from build123d import *
from build123d.topology import SkipClean

# Parameters (mm, degrees)
SKETCH1_W           = 50
SKETCH1_H           = 60
BOSS_EXTRUDE1_DEPTH = 12
SKETCH2_W           = 41
SKETCH2_H           = 4.2
CUT_EXTRUDE1_DEPTH  = 67.098411479
SKETCH3_W           = 12
SKETCH3_H           = 30
BOSS_EXTRUDE2_DEPTH = 42
SKETCH4_W           = 7.2
SKETCH4_H           = 20
CUT_EXTRUDE2_DEPTH  = 42.5
SKETCH5_R           = 2.55
CUT_EXTRUDE3_DEPTH  = 35
FILLET1_R           = 5
SKETCH6_R           = 2.55
CUT_EXTRUDE4_DEPTH  = 35
SKETCH7_R           = 2.9
BOSS_EXTRUDE3_DEPTH = 5


with BuildPart() as part:
    # Sketch1 → Boss-Extrude1 (new body)
    with BuildSketch(Plane.XY):
        Rectangle(SKETCH1_W, SKETCH1_H)
    extrude(amount=BOSS_EXTRUDE1_DEPTH)

    # Sketch2 → Cut-Extrude1 (cut, through all)
    with BuildSketch(Plane(origin=(0, 30, 0), x_dir=(1, 0, 0), z_dir=(0, 1, 0))):
        with Locations((0, -8.9)):
            Rectangle(SKETCH2_W, SKETCH2_H)
    extrude(amount=-CUT_EXTRUDE1_DEPTH, mode=Mode.SUBTRACT)

    # Sketch3 → Boss-Extrude2 (add)
    with BuildSketch(Plane.ZY.offset(25)):
        with Locations((6, -15)):
            Rectangle(SKETCH3_W, SKETCH3_H)
    boss_extrude2 = extrude(amount=BOSS_EXTRUDE2_DEPTH)

    # Sketch4 → Cut-Extrude2 (cut)
    with BuildSketch(Plane.ZY.offset(67)):
        with Locations((7.4, -15)):
            Rectangle(SKETCH4_W, SKETCH4_H)
    cut_extrude2 = extrude(amount=-CUT_EXTRUDE2_DEPTH, mode=Mode.SUBTRACT)

    # Sketch5 → Cut-Extrude3 (cut)
    with BuildSketch(Plane.XY.offset(12)):
        with Locations((-59.5, -14.995756269)):
            Circle(SKETCH5_R)
        with Locations((-51.2, -14.995756269)):
            Circle(SKETCH5_R)
        with Locations((-42.9, -14.995756269)):
            Circle(SKETCH5_R)
        with Locations((-34.6, -14.995756269)):
            Circle(SKETCH5_R)
    cut_extrude3 = extrude(amount=-CUT_EXTRUDE3_DEPTH, mode=Mode.SUBTRACT)

    # Mirror1: Boss-Extrude2, Cut-Extrude2, Cut-Extrude3 across plane
    add(boss_extrude2.mirror(Plane(origin=(0, 0, 0), x_dir=(0, 0, 1), z_dir=(1, 0, 0))))
    add(cut_extrude2.mirror(Plane(origin=(0, 0, 0), x_dir=(0, 0, 1), z_dir=(1, 0, 0))), mode=Mode.SUBTRACT)
    add(cut_extrude3.mirror(Plane(origin=(0, 0, 0), x_dir=(0, 0, 1), z_dir=(1, 0, 0))), mode=Mode.SUBTRACT)

    # Fillet1
    # the kernel refuses this fillet: 5 mm, written as the material it adds along each edge
    with BuildSketch(Plane(origin=(25, 0, 12), x_dir=(0, 1, 0), z_dir=(0, 0, -1))) as fillet1_piece_1:
        with BuildLine():
            CenterArc((FILLET1_R, FILLET1_R), FILLET1_R, 180, 90)
            Line((0, FILLET1_R), (0, 0))
            Line((0, 0), (FILLET1_R, 0))
        make_face()
    extrude(amount=12)
    with BuildSketch(Plane(origin=(-25, 0, 12), x_dir=(0, 1, 0), z_dir=(0, 0, -1))) as fillet1_piece_2:
        with BuildLine():
            CenterArc((FILLET1_R, -FILLET1_R), FILLET1_R, 90, 90)
            Line((0, -FILLET1_R), (0, 0))
            Line((0, 0), (FILLET1_R, 0))
        make_face()
    extrude(amount=12)
    # the kernel refuses this fillet: 5 mm, written as the material it takes off along each edge
    with BuildSketch(Plane(origin=(67, -30, -12.5), x_dir=(0, 1, 0), z_dir=(0, 0, 1)), Plane(origin=(-67, 0, 24.5), x_dir=(1, 0, 0), z_dir=(0, 0, -1)), Plane(origin=(25, 30, -12.5), x_dir=(-1, 0, 0), z_dir=(0, 0, 1))) as fillet1_2_piece_1:
        with BuildLine():
            CenterArc((FILLET1_R, FILLET1_R), FILLET1_R, 180, 90)
            Line((0, FILLET1_R), (0, 0))
            Line((0, 0), (FILLET1_R, 0))
        make_face()
    extrude(amount=37, mode=Mode.SUBTRACT)
    with BuildSketch(Plane(origin=(67, 0, 24.5), x_dir=(-1, 0, 0), z_dir=(0, 0, -1)), Plane(origin=(-67, -30, -12.5), x_dir=(0, 1, 0), z_dir=(0, 0, 1)), Plane(origin=(-25, 30, -12.5), x_dir=(1, 0, 0), z_dir=(0, 0, 1))) as fillet1_2_piece_2:
        with BuildLine():
            CenterArc((FILLET1_R, -FILLET1_R), FILLET1_R, 90, 90)
            Line((0, -FILLET1_R), (0, 0))
            Line((0, 0), (FILLET1_R, 0))
        make_face()
    extrude(amount=37, mode=Mode.SUBTRACT)

    # Sketch6 → Cut-Extrude4 (cut)
    with BuildSketch(Plane.XY.offset(12)):
        Circle(SKETCH6_R)
        with Locations((0, 10)):
            Circle(SKETCH6_R)
    extrude(amount=-CUT_EXTRUDE4_DEPTH, mode=Mode.SUBTRACT)

    # Sketch7 → Boss-Extrude3 (add)
    with SkipClean():  # the faces are left unmerged after this step: merging them gives an invalid solid
        with BuildSketch(Plane.XY.offset(12)):
            with BuildLine():
                ThreePointArc((-67, -25), (-65.535533906, -28.535533906), (-62, -30))
                Line((-62, -30), (62, -30))
                ThreePointArc((62, -30), (65.535533906, -28.535533906), (67, -25))
                Line((67, -25), (67, -5))
                ThreePointArc((67, -5), (65.535533906, -1.464466094), (62, 0))
                Line((62, 0), (30, 0))
                ThreePointArc((30, 0), (26.464466094, 1.464466094), (25, 5))
                Line((25, 5), (25, 25))
                ThreePointArc((25, 25), (23.535533906, 28.535533906), (20, 30))
                Line((20, 30), (-20, 30))
                ThreePointArc((-20, 30), (-23.535533906, 28.535533906), (-25, 25))
                Line((-25, 25), (-25, 5))
                ThreePointArc((-25, 5), (-26.464466094, 1.464466094), (-30, 0))
                Line((-30, 0), (-62, 0))
                ThreePointArc((-62, 0), (-65.535533906, -1.464466094), (-67, -5))
                Line((-67, -5), (-67, -25))
            make_face()
            with Locations((-59.5, -14.995756269)):
                Circle(SKETCH7_R, mode=Mode.SUBTRACT)
            with Locations((-51.2, -14.995756269)):
                Circle(SKETCH7_R, mode=Mode.SUBTRACT)
            with Locations((-42.9, -14.995756269)):
                Circle(SKETCH7_R, mode=Mode.SUBTRACT)
            with Locations((-34.6, -14.995756269)):
                Circle(SKETCH7_R, mode=Mode.SUBTRACT)
            with Locations((59.5, -14.995756269)):
                Circle(SKETCH7_R, mode=Mode.SUBTRACT)
            with Locations((51.2, -14.995756269)):
                Circle(SKETCH7_R, mode=Mode.SUBTRACT)
            with Locations((42.9, -14.995756269)):
                Circle(SKETCH7_R, mode=Mode.SUBTRACT)
            with Locations((34.6, -14.995756269)):
                Circle(SKETCH7_R, mode=Mode.SUBTRACT)
            with Locations((0, 10)):
                Circle(SKETCH7_R, mode=Mode.SUBTRACT)
            Circle(SKETCH7_R, mode=Mode.SUBTRACT)
        extrude(amount=BOSS_EXTRUDE3_DEPTH)


solid = part.part
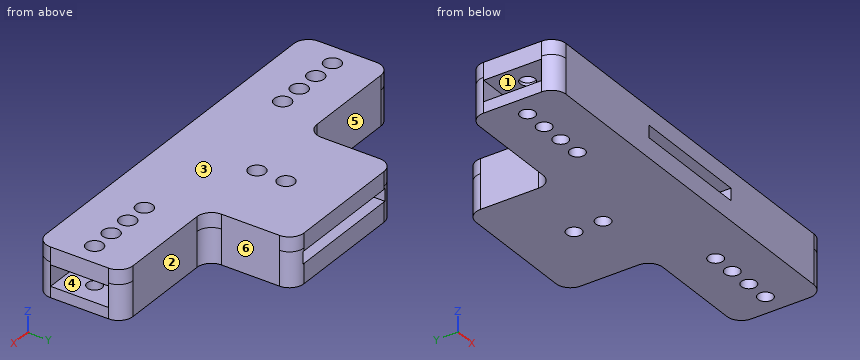
Could you check a few things on this model? Use its own coordinates, in mm. Face numbers are marked on the shaded views. A direction names the side the tool comes from. Give positions to 0.01 mm unless a question says otherwise; leave off trailing zeros. Loops run counter-clockwise (first coordinate to the right, second up) from the corner with the lowest first, then second, coordinate; pieces in that order, holes last. Notation, with made-up numbers: (20.25, 15) -> (70.25, 15) arc R22 ccw to (70.25, 48) -> close; hole circle Ø6 at (-25, 5). An arc over 180 degrees is marked (long way). Answer as CSV lines item,"result". Start each with the question number.
(1) Which directions (+Z, -Z, +X, -X, +Y, -Y) give clear straight access to the entire face, cutting with the end or side of a thin tool? Please do the marked faces 4, 5 and 6.
(2) I need wall thicknesses on probe 1 along Y at (x, z) = (0, 2.75); probe 2 along Y at (x, z) = (0, 14.9); probe 3 along X at (y, z) = (-22.5, 10.25). Which ranges of each line are inside material? Lowest first, please.
(3) We'd pull the mould along Y, two halves only. Please class the marked faces 1, 2 and 3: released by +Y, released by -Y, zero draft, split by the parting line, or undercut.
(4) I'm going to push flat-ended pins straight in: pin 1 Ø8 at (x, z) = (-38.5, 6.5) entering from +Y; pin 2 Ø5 at (y, z) = (-17, 6.5) entering from +X; pin 3 Ø3.5 at (y, z) = (-15.5, 6.5) entering from -X. Where does each tip first touch, or does it pass through?
(5) If we section it at C-C on x = 0: Count the separate pieces of the cut face and the enclosed holes in it, then the cut area to 3 significant figures.
(6) If we section it at A-A on z = 9.25: Write out the boundary of the cut face in (x, y), then the cut area to 3 significant figures.
(7) If we section it at D-D on y = 20: Write out the boundary of the cut face in (x, z), then the cut area to 3 significant figures.
(8) If we section it at B-B on x = -34.6: Write out the boundary of the cut face in (y, z).
Computed:
1,face 4,"+X"
1,face 5,"+Z, -Z, -X, +Y"
1,face 6,"+Z, -Z, +X, +Y"
2,probe 1,"y = -30 to -2.55, 2.55 to 7.45, 12.55 to 30"
2,probe 2,"y = -30 to -2.9, 2.9 to 7.1, 12.9 to 30"
2,probe 3,"x = -24.5 to -20.5, 20.5 to 24.5"
3,face 1,"undercut"
3,face 2,"released by +Y"
3,face 3,"zero draft"
4,pin 1,"stops at y = 0"
4,pin 2,"stops at x = 24.5"
4,pin 3,"stops at x = -24.5"
5,separate pieces,"6"
5,enclosed holes,"0"
5,area,"630 mm2"
6,outline,"(-67, -25) arc R5 ccw to (-62, -30) -> (-20.5, -30) -> (-20.5, 29.97) arc R5 ccw to (-25, 25) -> (-25, 5) arc R5 cw to (-30, 0) -> (-62, 0) arc R5 ccw to (-67, -5) -> (-24.5, -5) -> (-24.5, -25) -> close; (20.5, -30) -> (62, -30) arc R5 ccw to (67, -25) -> (24.5, -25) -> (24.5, -5) -> (67, -5) arc R5 ccw to (62, 0) -> (30, 0) arc R5 cw to (25, 5) -> (25, 25) arc R5 ccw to (20.5, 29.97) -> close"
6,area,"1,340 mm2"
7,outline,"(-25, 0) -> (25, 0) -> (25, 17) -> (-25, 17) -> close; hole (-20.5, 6.8) -> (20.5, 6.8) -> (20.5, 11) -> (-20.5, 11) -> close"
7,area,"678 mm2"
8,outline,"(-30, 0) -> (-17.55, 0) -> (-17.55, 3.8) -> (-25, 3.8) -> (-25, 11) -> (-17.55, 11) -> (-17.55, 12) -> (-17.9, 12) -> (-17.9, 17) -> (-30, 17) -> close; (-12.45, 0) -> (0, 0) -> (0, 17) -> (-12.1, 17) -> (-12.1, 12) -> (-12.45, 12) -> (-12.45, 11) -> (-5, 11) -> (-5, 3.8) -> (-12.45, 3.8) -> close"
